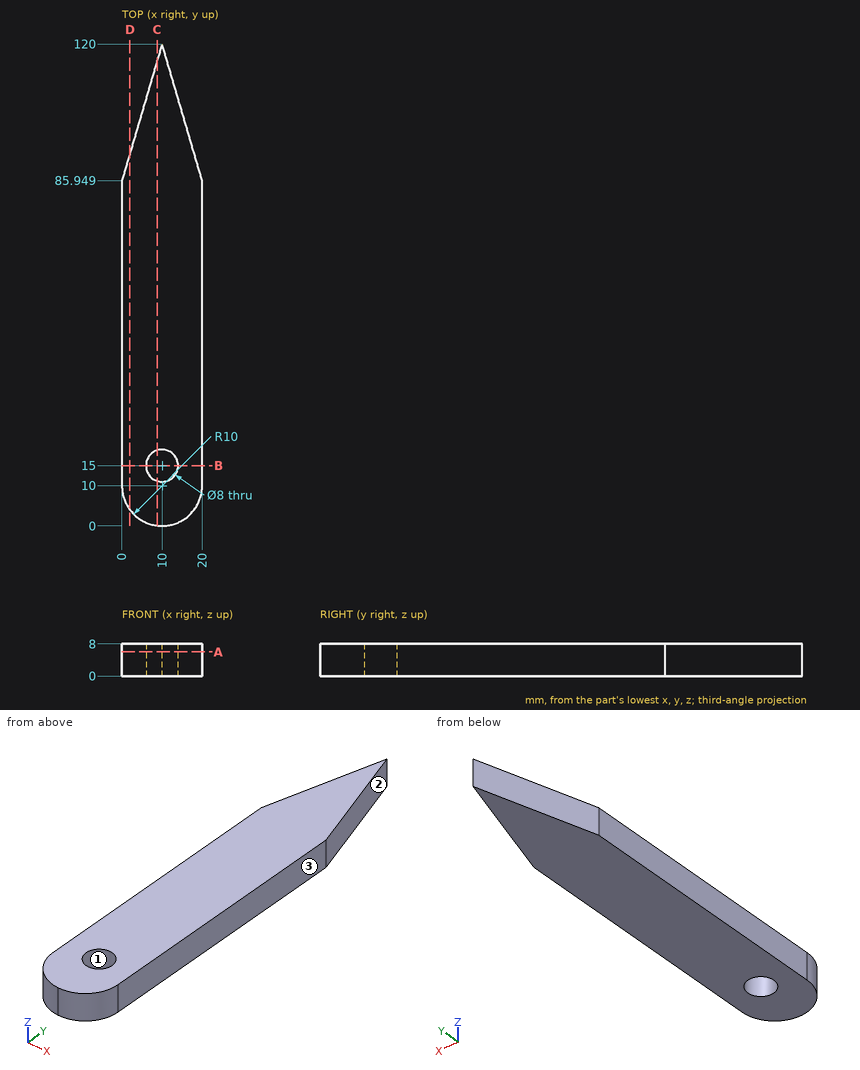
Geometry check sheet. Reference: drawing and pictorial views, mm from the part's lowest x, y, z. Give positions to 0.01 mm unless a question says otherwise; leave off trailing zeros. Order: outer loops, then holes, each group sorted by start corner. A loop starts at its lowest first (then second) coordinate and runs counter-clockwise, first axis right, second up.
1. Section check C-C, the plane x = 8.75. Enter the section's corners in (y, z).
2. Gauge pin test, flat ends, axial feed: pin 1 Ø4 at (y, z) = (92.5, 4) entering from +X; pin 2 Ø1 at (y, z) = (107, 4.5) entering from +X (1 decimal). Record the tip position at first contact, or that the pin passes through.
3. Section check B-B, the plane y = 15. Enter the section's corners in (x, z), and give its area (3 significant figures).
4. Section check A-A, the plane z = 6. Enter the section's corners in (x, y).
5. Thickness scan on L1, parallel to X at y = 114, z = 2.75; L2, parallel to X at y = 7, z = 5.5. Record the ranges inside material, lowest first.
6. Release check for a two-part mould opening along Y. For the marked faces 1, 2 and 3 record: pulls with the +Y half, pulls with the -Y half, needs draft (parallel to the pull), parting line crosses it, or undercut.
7. Section check D-D, the plane x = 2. Enter the section's corners in (y, z).
Values follow:
1. outline: (0.08, 0) - (11.2, 0) - (11.2, 8) - (0.08, 8) - close; (18.8, 0) - (115.74, 0) - (115.74, 8) - (18.8, 8) - close
2. pin 1: stops at x = 18.66
2. pin 2: stops at x = 14
3. outline: (0, 0) - (6, 0) - (6, 8) - (0, 8) - close; (14, 0) - (20, 0) - (20, 8) - (14, 8) - close
3. area: 96.0 mm2
4. outline: (0, 10) arc R10 ccw to (10, 0) arc R10 ccw to (20, 10) - (20, 85.95) - (10, 120) - (0, 85.95) - close; hole circle Ø8 at (10, 15)
5. L1: x = 8.24 to 11.76
5. L2: x = 0.46 to 19.54
6. face 1: undercut
6. face 2: pulls with the +Y half
6. face 3: needs draft
7. outline: (4, 0) - (92.76, 0) - (92.76, 8) - (4, 8) - close
